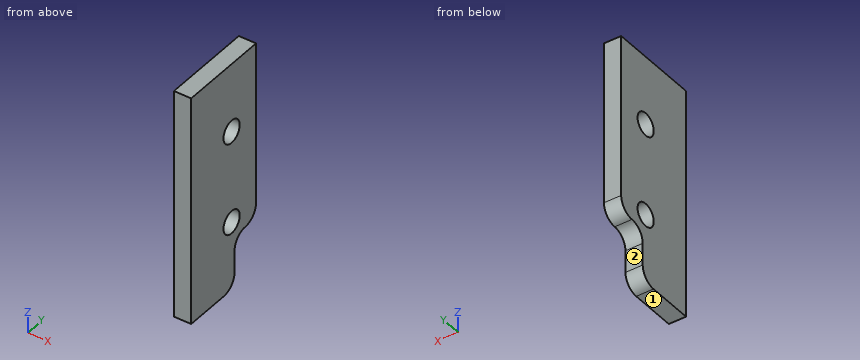
from build123d import *

# Parameters (mm, degrees)
SKETCH1_W           = 42.418
SKETCH1_H           = 16.8402
BOSS_EXTRUDE1_DEPTH = 3.175
SKETCH3_R           = 2.1
CUT_EXTRUDE1_DEPTH  = 24.039105669
SKETCH4_W           = 9.652
SKETCH4_H           = 5.588
CUT_EXTRUDE2_DEPTH  = 24.039105669
FILLET1_R           = 2.794


with BuildPart() as part:
    # Sketch1 → Boss-Extrude1 (new body)
    with BuildSketch(Plane(origin=(0, 0, 0), x_dir=(0, 0, -1), z_dir=(1, 0, 0))):
        Rectangle(SKETCH1_W, SKETCH1_H)
    extrude(amount=BOSS_EXTRUDE1_DEPTH)

    # Sketch3 → Cut-Extrude1 (cut, through all)
    with BuildSketch(Plane(origin=(3.175, 0, 0), x_dir=(0, 0, -1), z_dir=(1, 0, 0))):
        with Locations((-8.509, 2.0701)):
            Circle(SKETCH3_R)
        with Locations((8.509, 2.0701)):
            Circle(SKETCH3_R)
    extrude(amount=-CUT_EXTRUDE1_DEPTH, mode=Mode.SUBTRACT)

    # Sketch4 → Cut-Extrude2 (cut, through all)
    with BuildSketch(Plane(origin=(3.175, 0, 0), x_dir=(0, 0, -1), z_dir=(1, 0, 0))):
        with Locations((16.383, 5.6261)):
            Rectangle(SKETCH4_W, SKETCH4_H)
    extrude(amount=-CUT_EXTRUDE2_DEPTH, mode=Mode.SUBTRACT)

    # Fillet1
    fillet1_edges = [part.edges().sort_by_distance(p)[0] for p in [
        (1.5875, 2.8321, -21.209),
        (1.5875, 8.4201, -11.557),
        (1.5875, 2.8321, -11.557),
    ]]
    fillet(fillet1_edges, radius=FILLET1_R - 0.0001)  # a hair under: the kernel refuses the full size


solid = part.part
Source: CAD feature listing. Evaluate the final solid. Frame: model axes, mm. Face numbers are marked on the shaded views. A direction names the side the tool comes from. Give positions to 0.01 mm unless a question says otherwise; leave off trailing zeros. Loops run counter-clockwise (first coordinate to the right, second up) from the corner with the lowest first, then second, coordinate; pieces in that order, holes last. Notation, with made-up numbers: (74, -4) -> (122, -4) arc R22 ccw to (122, 25) -> close; hole circle Ø4 at (-24.75, 8.25). An arc over 180 degrees is marked (long way). Use a Markdown table: item, result. Add a question column.
1) First-contact query: pin 1 (5 mm diameter, centred on y = -3, z = 14, fed in from -X); pin 2 (1.5 mm diameter, centred on x = 1.5, z = -16, fed in from +Y). Flat tips, straight axial feed; report the tip coordinate or a pass-through.
2) Section query A-A, the plane z = -9.5. Return the cut outline in (x, y) (3 decimals).
3) Line query: line 1 along Z through (x, y) = (1.1, 1.5); line 2 along Z through (x, y) = (1, 3.75); line 3 along Y through (x, z) = (0.3, -15.5). Output: solid intervals per line, ascending. Write a range as [from, to].
4) Section query D-D, the plane y = 7.75. Return the cut outline in (x, z) (3 decimals), then the cut area to 3 significant figures.
5) Section query B-B, the plane y = 0.5. Return the cut outline in (x, z) (3 decimals).
6) Reachability of the marked faces 1 and 2 from +Z, -Z, +X, -X, +Y, -Y: full face, straight path, thin tool, end or side. Return the list, or none.
7) Section query C-C, the plane x = 1.1. Count the separate pieces of the cut face and the enclosed holes in it, then the cut area to 3 significant figures.
Numbers:
| question | item | result |
|---|---|---|
| 1 | pin 1 | stops at x = 0 |
| 1 | pin 2 | stops at y = 2.83 |
| 2 | outline | (0, -8.42) -> (3.175, -8.42) -> (3.175, 0.219) -> (0, 0.219) -> close; (0, 3.922) -> (3.175, 3.922) -> (3.175, 8.321) -> (0, 8.321) -> close |
| 3 | line 1 | z = [-20.8, -10.53], [-6.49, 6.49], [10.53, 21.21] |
| 3 | line 2 | z = [-12.28, -9.77], [-7.25, 7.25], [9.77, 21.21] |
| 3 | line 3 | y = [-8.42, 2.83] |
| 4 | outline | (0, -10.578) -> (3.175, -10.578) -> (3.175, 21.209) -> (0, 21.209) -> close |
| 4 | area | 101 mm2 |
| 5 | outline | (0, -21.171) -> (3.175, -21.171) -> (3.175, -9.904) -> (0, -9.904) -> close; (0, -7.114) -> (3.175, -7.114) -> (3.175, 7.114) -> (0, 7.114) -> close; (0, 9.904) -> (3.175, 9.904) -> (3.175, 21.209) -> (0, 21.209) -> close |
| 6 | face 1 | -Z, +X, -X, +Y, -Y |
| 6 | face 2 | -Z, +X, -X, +Y |
| 7 | separate pieces | 1 |
| 7 | enclosed holes | 2 |
| 7 | area | 631 mm2 |
